Here's how the part is built. I have some questions about the finished solid (model axes, mm). Face numbers are marked on the shaded views. A direction names the side the tool comes from. Round coordinates to 2 decimals unless told otherwise and drop trailing zeros. Order: outer loops, then holes, each group sorted by start corner. A loop starts at its lowest first (then second) coordinate and runs counter-clockwise, first axis right, second up. Notation, with made-up numbers: M -1,1.25 L 41,1.25 A22 cw 41,14.25 Z; hole C 47.25,47.25 d3. An arc over 180 degrees is marked long. Answer as CSV lines item,"result". Start each with the question number.
```python
from build123d import *

# Parameters (mm, degrees)
SKETCH_1_W          = 26.5
SKETCH_1_H          = 17.5
EXTRUDE_1_DEPTH     = 15.1
SKETCH_2_W          = 5.4
SKETCH_2_H          = 4.2
EXTRUDE_2_DEPTH     = 3.5
SKETCH_3_W          = 2.08
SKETCH_3_H          = 2.08
SKETCH_3_W_2        = 3.88
SKETCH_3_H_2        = 3.88
CUT_EXTRUDE_1_DEPTH = 3.88
SKETCH_4_W          = 8
SKETCH_4_H          = 2
CUT_EXTRUDE_2_DEPTH = 1
FILLET_1_R          = 1.5
FILLET_2_R          = 1
FILLET_3_R          = 0.5
FILLET_4_R          = 0.2
SKETCH_5_W          = 16
SKETCH_5_H          = 2.83
EXTRUDE_3_DEPTH     = 0.5


with BuildPart() as part:
    # 草图1 → 凸台-拉伸1 (new body)
    with BuildSketch(Plane(origin=(0, 0, 0), x_dir=(1, 0, 0), z_dir=(0, 1, 0))):
        Rectangle(SKETCH_1_W, SKETCH_1_H)
    extrude(amount=EXTRUDE_1_DEPTH)

    # 草图2 → 凸台-拉伸2 (add)
    with BuildSketch(Plane(origin=(13.25, 0, 0), x_dir=(0, 0, -1), z_dir=(1, 0, 0))):
        with Locations((6.05, 2.1)):
            Rectangle(SKETCH_2_W, SKETCH_2_H)
    extrude(amount=EXTRUDE_2_DEPTH)

    # 草图3 → 切除-拉伸1 (cut)
    with BuildSketch(Plane(origin=(0, 15.1, 0), x_dir=(1, 0, 0), z_dir=(0, 1, 0))):
        with Locations((-12.21, 7.71)):
            Rectangle(SKETCH_3_W, SKETCH_3_H)
        with Locations((-11.31, -6.81)):
            Rectangle(SKETCH_3_W_2, SKETCH_3_H_2)
        with Locations((11.31, -6.81)):
            Rectangle(SKETCH_3_W_2, SKETCH_3_H_2)
        with Locations((12.21, 7.71)):
            Rectangle(SKETCH_3_W, SKETCH_3_H)
    extrude(amount=-CUT_EXTRUDE_1_DEPTH, mode=Mode.SUBTRACT)

    # 草图4 → 切除-拉伸2 (cut)
    with BuildSketch(Plane.XZ):
        with Locations((0, 8.75)):
            Rectangle(SKETCH_4_W, SKETCH_4_H)
    extrude(amount=-CUT_EXTRUDE_2_DEPTH, mode=Mode.SUBTRACT)

    # 圆角1
    fillet_1_edges = [part.edges().sort_by_distance(p)[0] for p in [
        (13.25, 5.61, 8.75),
        (-13.25, 5.61, 8.75),
        (-13.25, 5.61, -8.75),
        (13.25, 7.71, -8.75),
    ]]
    fillet(fillet_1_edges, radius=FILLET_1_R)

    # 圆角2
    fillet_2_edges = [part.edges().sort_by_distance(p)[0] for p in [
        (9.37, 13.16, 4.87),
        (-9.37, 13.16, 4.87),
    ]]
    fillet(fillet_2_edges, radius=FILLET_2_R)

    # 圆角3
    fillet_3_edges = [part.edges().sort_by_distance(p)[0] for p in [
        (11.17, 13.16, -6.67),
        (-11.17, 13.16, -6.67),
    ]]
    fillet(fillet_3_edges, radius=FILLET_3_R)

    # 圆角4
    fillet_4_edges = [part.edges().sort_by_distance(p)[0] for p in [
        (9.37, 15.1, 7.31),
        (-11.81, 15.1, 4.87),
        (9.662893219, 15.1, 5.162893219),
        (-9.662893219, 15.1, 5.162893219),
        (-11.17, 15.1, -7.96),
        (12.46, 15.1, -6.67),
        (-11.316446609, 15.1, -6.816446609),
        (11.316446609, 15.1, -6.816446609),
        (14.25, 4.2, -8.75),
        (15, 4.2, -3.35),
        (13.25, 15.1, -0.9),
        (0, 15.1, -8.75),
        (-13.25, 15.1, -0.9),
        (0, 15.1, 8.75),
        (11.17, 15.1, -7.96),
        (11.81, 15.1, 4.87),
        (-9.37, 15.1, 7.31),
        (-12.46, 15.1, -6.67),
    ]]
    fillet(fillet_4_edges, radius=FILLET_4_R)

    # 草图5 → 凸台-拉伸3 (add)
    with BuildSketch(Plane(origin=(0, 15.1, 0), x_dir=(1, 0, 0), z_dir=(0, 1, 0))):
        with Locations((0, 1.865)):
            Rectangle(SKETCH_5_W, SKETCH_5_H)
        with Locations((0, -6.165)):
            Rectangle(SKETCH_5_W, SKETCH_5_H)
    extrude(amount=EXTRUDE_3_DEPTH)


solid = part.part
```
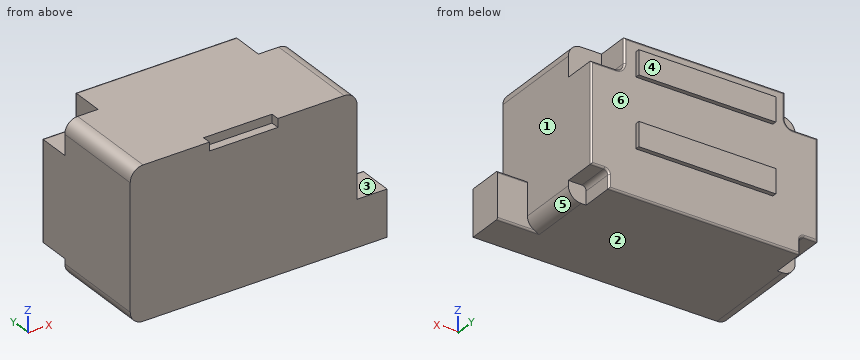
Item 1: If I drill on line 1 along Y through (x, z) = (15, -6); line 2 along Y through (x, z) = (0, 4); line 3 along X through (y, z) = (2.5, 5), over which ranges is the centre line in solid material (lowest first)?
Item 2: For P1, Ø0.6, axis at y = 15.5, z = 5.5, coming from the -X side; P2, Ø0.9, axis at y = 13, z = 7.5, coming from the +X side; P3, Ø1.2, axis at x = 10.5, z = 6.5, coming from the +Y side, each with a flat end and sliding along its axis, tell me the tip position at first contact or that it passes through.
Item 3: If we section it at A-A on y = 14: Please give me the cut outline in (x, z), and give its area (3 significant figures).
Item 4: Which directions (+Z, -Z, +X, -X, +Y, -Y) give clear straight access to the entire face, cutting with the end or side of a thin tool? Please do the marked faces 1, 2 and 3.
Item 5: We'd pull the mould along Z, two halves only. Please class the marked faces 4, 5 and 6: pulls with the +Z half, pulls with the -Z half, needs draft (parallel to the pull), parting line crosses it, or undercut.
Item 6: If we section it at D-D on x = 14.5: Please give me the cut outline in (y, z), and give its area (3 significant figures).
Item 7: If we section it at B-B on x = -6: Please give me the cut outline in (y, z).
Item 8: If we section it at C-C on z = -5.75: Please give me the cut outline in (x, y), and give its area (3 significant figures).
Geometry says:
1,line 1,"0 to 4.2"
1,line 2,"0 to 15.1"
1,line 3,"-13.25 to 13.25"
2,P1,"x = -8"
2,P2,"x = 9.37"
2,P3,"y = 11.22"
3,outline,"M -13.25,-6.67 L -11.67,-6.67 A0.5 cw -11.17,-7.17 L -11.17,-8.75 L 11.17,-8.75 L 11.17,-7.17 A0.5 cw 11.67,-6.67 L 13.25,-6.67 L 13.25,4.87 L 10.37,4.87 A1 cw 9.37,5.87 L 9.37,8.75 L -9.37,8.75 L -9.37,5.87 A1 cw -10.37,4.87 L -13.25,4.87 Z"
3,area,"426 mm²"
4,face 1,"+Z, +X, +Y"
4,face 2,"-Z, +X, -X, +Y, -Y"
4,face 3,"+Z, +X, +Y, -Y"
5,face 4,"needs draft"
5,face 5,"pulls with the -Z half"
5,face 6,"undercut"
6,outline,"M 0,-8.75 L 4,-8.75 A0.2 ccw 4.2,-8.55 L 4.2,-3.55 A0.2 ccw 4,-3.35 L 0,-3.35 Z"
6,area,"22.7 mm²"
7,outline,"M 0,-8.75 L 14.9,-8.75 A0.2 ccw 15.1,-8.55 L 15.1,-3.28 L 15.6,-3.28 L 15.6,-0.45 L 15.1,-0.45 L 15.1,4.75 L 15.6,4.75 L 15.6,7.58 L 15.1,7.58 L 15.1,8.55 A0.2 ccw 14.9,8.75 L 0,8.75 Z"
8,outline,"M -13.25,0 L 16.75,0 L 16.75,4.2 L 13.25,4.2 L 13.25,14.9 A0.2 ccw 13.05,15.1 L -13.05,15.1 A0.2 ccw -13.25,14.9 Z"
8,area,"415 mm²"
